```python
from build123d import *

# Parameters (mm, degrees)
IZIM1_R                     = 11.075
IZIM1_R_2                   = 2.6
Y_KSEKLIK_EKSTR_ZYON2_DEPTH = 6


with BuildPart() as part:
    # Çizim1 → Yükseklik-Ekstrüzyon2 (new body)
    with BuildSketch(Plane.XY):
        with BuildLine():
            Line((-56.410377678, 29.652139902), (-56.410377678, -30.347860098))
            Line((-56.410377678, -30.347860098), (13.589622322, -30.347860098))
            Line((13.589622322, -30.347860098), (13.589622322, 29.652139902))
            ThreePointArc((13.589622322, 29.652139902), (-21.410377678, 64.652139902), (-56.410377678, 29.652139902))
        make_face()
        with Locations((-21.410377678, 49.652139902)):
            Circle(IZIM1_R, mode=Mode.SUBTRACT)
        with Locations((-50.410377678, -24.347860098)):
            Circle(IZIM1_R_2, mode=Mode.SUBTRACT)
        with Locations((7.589622322, -24.347860098)):
            Circle(IZIM1_R_2, mode=Mode.SUBTRACT)
        with Locations((-50.410377678, -4.347860098)):
            Circle(IZIM1_R_2, mode=Mode.SUBTRACT)
        with Locations((7.589622322, -4.347860098)):
            Circle(IZIM1_R_2, mode=Mode.SUBTRACT)
        with BuildLine():
            Line((-12.160377678, 4.652139902), (-12.160377678, -5.347860098))
            ThreePointArc((-12.160377678, -5.347860098), (-21.410377678, -14.597860098), (-30.660377678, -5.347860098))
            Line((-30.660377678, -5.347860098), (-30.660377678, 4.652139902))
            ThreePointArc((-30.660377678, 4.652139902), (-21.410377678, 13.902139902), (-12.160377678, 4.652139902))
        make_face(mode=Mode.SUBTRACT)
        with BuildLine():
            Line((-33.810377678, 4.652139902), (-33.810377678, -5.347860098))
            ThreePointArc((-33.810377678, -5.347860098), (-35.910377678, -7.447860098), (-38.010377678, -5.347860098))
            Line((-38.010377678, -5.347860098), (-38.010377678, 4.652139902))
            ThreePointArc((-38.010377678, 4.652139902), (-35.910377678, 6.752139902), (-33.810377678, 4.652139902))
        make_face(mode=Mode.SUBTRACT)
        with BuildLine():
            Line((-4.810377678, 4.652139902), (-4.810377678, -5.347860098))
            ThreePointArc((-4.810377678, -5.347860098), (-6.910377678, -7.447860098), (-9.010377678, -5.347860098))
            Line((-9.010377678, -5.347860098), (-9.010377678, 4.652139902))
            ThreePointArc((-9.010377678, 4.652139902), (-6.910377678, 6.752139902), (-4.810377678, 4.652139902))
        make_face(mode=Mode.SUBTRACT)
    extrude(amount=Y_KSEKLIK_EKSTR_ZYON2_DEPTH)


solid = part.part
```
Check sheet for the modelled part. Datum: model origin and axes. Units: mm. A direction names the side the tool comes from. Round coordinates to 2 decimals unless told otherwise and drop trailing zeros. Write each loop counter-clockwise with the first axis right and the second up, starting at its lowest first coordinate (ties: lowest second). Pieces come first, ordered by that corner, then holes. Notation, with made-up numbers: M -34,17 L 8,17 A20 cw 8,48 Z; hole C 9.5,31.5 d8. An arc over 180 degrees is marked long. Write item = value, one per line. Start each with the question number.
1. Tool access check on faces 1 (the flat face through (-9.01, 0, 3)), 2 (the flat face through (-22, 18, 6)). Record the directions out of +Z, -Z, +X, -X, +Y, -Y that give a thin tool (end or side, any length) a straight path to the whole face; none if there is none.
2. Section check D-D, the plane y = -13. Record the cut outline in (x, z).
3. Release check for a two-part mould opening along X. For faces 3 (the cylindrical face through (-35.96, 6.75, 2.96)), 4 (the flat face through (-33.81, 0, 3)), 5 (the flat face through (-22, 18, 0)), 6 (the flat face through (13.59, -1, 3)) record: pulls with the +X half, pulls with the -X half, needs draft (parallel to the pull), parting line crosses it, or undercut.
4. Section check B-B, the plane x = -21.5. Record the cut outline in (y, z), then the cut area to 3 significant figures.
5. Scan lines: line 1 (X direction, y = 2, z = 0.75); line 2 (Y direction, x = -22, z = 0.35); line 3 (Y direction, x = -24, z = 2.6). Record each from-to range of solid material in increasing order. Write a range as [from, to].
6. Section check C-C, the plane z = 4.85. State how many separate pieces and enclosed holes the cut face has, then the cut area to 3 significant figures.
7. Gauge pin test, flat ends, axial feed: pin 1 (3 mm diameter, centred on x = -6.5, z = 1, fed in from +Y); pin 2 (20 mm diameter, centred on x = -21.41, y = 49.65, fed in from -Z). Record the tip position at first contact, or that the pin passes through.
8. Section check A-A, the plane y = 42.5. Record the cut outline in (x, z).
Results found:
q1.face_1 = +Z, -Z
q1.face_2 = +Z, +X, -X, +Y, -Y
q2.outline = M -56.41,0 L -26.61,0 L -26.61,6 L -56.41,6 Z; M -16.21,0 L 13.59,0 L 13.59,6 L -16.21,6 Z
q3.face_3 = undercut
q3.face_4 = undercut
q3.face_5 = needs draft
q3.face_6 = pulls with the +X half
q4.outline = M -30.35,0 L -14.6,0 L -14.6,6 L -30.35,6 Z; M 13.9,0 L 38.58,0 L 38.58,6 L 13.9,6 Z; M 60.73,0 L 64.65,0 L 64.65,6 L 60.73,6 Z
q4.area = 266 mm^2
q5.line_1 = [-56.41, -38.01], [-33.81, -30.66], [-12.16, -9.01], [-4.81, 13.59]
q5.line_2 = [-30.35, -14.58], [13.88, 38.59], [60.71, 64.65]
q5.line_3 = [-30.35, -14.23], [13.53, 38.88], [60.42, 64.56]
q6.separate_pieces = 1
q6.enclosed_holes = 8
q6.area = 5,090 mm^2
q7.pin_1 = 61.98
q7.pin_2 = through
q8.outline = M -53.97,0 L -29.87,0 L -29.87,6 L -53.97,6 Z; M -12.95,0 L 11.15,0 L 11.15,6 L -12.95,6 Z
